from build123d import *

# Parameters (mm, degrees)
SKETCH_1_R          = 3.6
SKETCH_1_R_2        = 1.5
EXTRUDE_1_DEPTH     = 2.5
CUT_EXTRUDE_START   = -1.9
SKETCH_2_R          = 3.6
SKETCH_2_R_2        = 3
CUT_EXTRUDE_1_DEPTH = 1.9
CHAMFER_1_SIZE      = 0.1


with BuildPart() as part:
    # 草图1 → 凸台-拉伸1 (new body)
    with BuildSketch(Plane(origin=(0, 0, 0), x_dir=(1, 0, 0), z_dir=(0, 1, 0))):
        with Locations(Location((0, 0, 0), (0, 0, 270))):
            Circle(SKETCH_1_R)
        with Locations(Location((0, 0, 0), (0, 0, 270))):
            Circle(SKETCH_1_R_2, mode=Mode.SUBTRACT)
    extrude(amount=EXTRUDE_1_DEPTH)

    # 草图2 → 切除-拉伸1 (cut)
    with BuildSketch(Plane(origin=(0, 2.5, 0), x_dir=(1, 0, 0), z_dir=(0, 1, 0)).offset(CUT_EXTRUDE_START)):
        with Locations(Location((0, 0, 0), (0, 0, 270))):
            Circle(SKETCH_2_R)
        with Locations(Location((0, 0, 0), (0, 0, 270))):
            Circle(SKETCH_2_R_2, mode=Mode.SUBTRACT)
    extrude(amount=CUT_EXTRUDE_1_DEPTH, mode=Mode.SUBTRACT)

    # 倒角1
    chamfer_1_edges = [part.edges().sort_by_distance(p)[0] for p in [
        (0, 0.6, -3.6),
        (0, 2.5, -3),
        (0, 0, -3.6),
    ]]
    chamfer(chamfer_1_edges, length=CHAMFER_1_SIZE)


solid = part.part
Geometry check sheet. Reference: the model listing, model coordinates, mm. Give positions to 0.01 mm unless a question says otherwise; leave off trailing zeros. Loops run counter-clockwise (first coordinate to the right, second up) from the corner with the lowest first, then second, coordinate; pieces in that order, holes last. Notation, with made-up numbers: (25, 78) -> (53, 78) arc R24 ccw to (53, 104) -> close; hole circle Ø2 at (-28.75, 22). An arc over 180 degrees is marked (long way). Answer in a Markdown table with one row per item. Add a question column.
1) Draft check along Z on faces 1 (the face through (0.45, 1.23, 1.43)), 2 (the face through (0.9, 1.49, 2.86)), 3 (the face through (1, 0.6, 3)). Enter one of: pulls with the +Z half, pulls with the -Z half, needs draft (parallel to the pull), parting line crosses it, or undercut.
2) Cross-section at B-B on y = 1. Record the boundary of the cut face in (x, z).
3) Material ranges on probe 1 along X at (y, z) = (0.8, 0); probe 2 along Y at (x, z) = (2.75, 1.5); probe 3 along X at (y, z) = (2.35, -0.5), recorded low to high. Write a range as from..to.
4) Gauge pin test, flat end, axial feed: P1, Ø1, axis at x = 1.5, z = 1, coming from the -Y side. Record the tip position at first contact, or that the pin passes through.
5) Cross-section at C-C on y = 0.2. Record the boundary of the cut face in (x, z), and give its area (3 significant figures).
6) Cross-section at A-A on z = 0. Record the boundary of the cut face in (x, y).
Outcome:
| question | item | result |
|---|---|---|
| 1 | face 1 | undercut |
| 1 | face 2 | parting line crosses it |
| 1 | face 3 | needs draft |
| 2 | outline | circle Ø6 at (0, 0); hole circle Ø3 at (0, 0) |
| 3 | probe 1 | x = -3..-1.5, 1.5..3 |
| 3 | probe 2 | y = 0..0.6 |
| 3 | probe 3 | x = -2.96..-1.41, 1.41..2.96 |
| 4 | P1 | stops at y = 0 |
| 5 | outline | circle Ø7.2 at (0, 0); hole circle Ø3 at (0, 0) |
| 5 | area | 33.6 mm^2 |
| 6 | outline | (-3.6, 0.1) -> (-3.5, 0) -> (-1.5, 0) -> (-1.5, 2.5) -> (-2.9, 2.5) -> (-3, 2.4) -> (-3, 0.6) -> (-3.5, 0.6) -> (-3.6, 0.5) -> close; (1.5, 0) -> (3.5, 0) -> (3.6, 0.1) -> (3.6, 0.5) -> (3.5, 0.6) -> (3, 0.6) -> (3, 2.4) -> (2.9, 2.5) -> (1.5, 2.5) -> close |
